```python
from build123d import *


with BuildPart() as part:
    # Sweep1: sweep along a path in Sketch2
    with BuildLine(Plane.XY) as sweep1_path:
        Line((3.4, -33.829572862), (-194.6, -53.729321604))
        ThreePointArc((-194.6, -53.729321604), (-254, 0), (-194.6, 53.729321604))
        Line((-194.6, 53.729321604), (3.4, 33.829572862))
        ThreePointArc((3.4, 33.829572862), (34, 0), (3.4, -33.829572862))
    # Sketch4 → Sweep1 (sweep)
    with BuildSketch(Plane(origin=(0, 0, 0), x_dir=(0, 0, -1), z_dir=(1, 0, 0))):
        Polygon((0, 34.171285719), (6.035, 34.171285719), (9.499101615, 40.171285719), (-9.499101615, 40.171285719), (-6.035, 34.171285719), align=None)
    sweep(path=sweep1_path.line)


solid = part.part
```
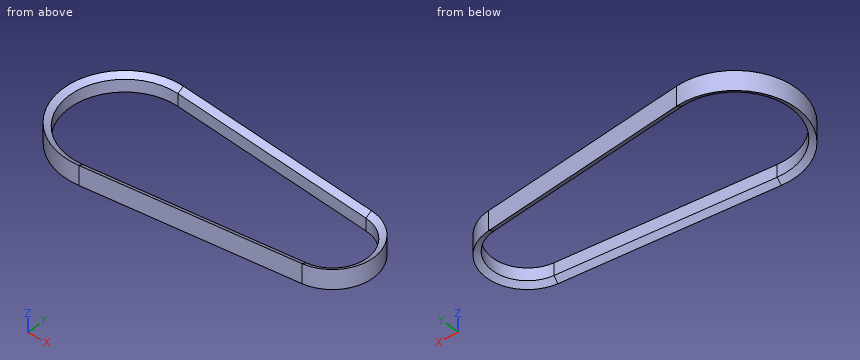
Source: CAD feature listing. Evaluate the final solid. Frame: model axes, mm. Round coordinates to 2 decimals unless told otherwise and drop trailing zeros. Order: outer loops, then holes, each group sorted by start corner. A loop starts at its lowest first (then second) coordinate and runs counter-clockwise, first axis right, second up. Notation, with made-up numbers: (32.25, 74.5) -> (63.25, 74.5) arc R18 ccw to (63.25, 88.5) -> close; hole circle Ø4 at (47.25, 25.5). An arc over 180 degrees is marked (long way). One line per item, written item: value. Start each with the question number.
Q1. Material intervals for probe 1 along Y at (x, z) = (-200, 0); probe 2 along X at (y, z) = (-30, -5); probe 3 along X at (y, z) = (2, 8.75), sorted ascending.
Q2. Section query A-A (z = -2.75). Return the cut outline in (x, y), plus the area to 3 significant figures.
Q3. Pin query (flat end, axial travel): pin 1 (1 mm diameter, centred on x = -15, z = 3.5, fed in from +Y); pin 2 (10 mm diameter, centred on x = 2.5, z = 7.5, fed in from +Y); pin 3 (1 mm diameter, centred on x = -99.5, y = 47, fed in from +Z). Return the tip coordinate at first contact, or that it passes through.
Q4. Section query B-B (x = -39.5). Return the cut outline in (y, z) (3 decimals).
Findings below:
1. probe 1: -59.97 to -54, 54 to 59.97
1. probe 2: -251.93 to -244.9, 16 to 26.42
1. probe 3: -259.94 to -258.65, 38.63 to 39.92
2. outline: (-194.6, 59.73) arc R59.97 ccw (long way) to (-193.41, -59.61) -> (4.59, -39.71) arc R39.97 ccw to (3.4, 39.83) -> close; hole (-194.6, -53.73) -> (3.4, -33.83) arc R34 ccw to (3.4, 33.83) -> (-194.6, 53.73) arc R54 ccw (long way) to start
2. area: 4,160 mm²
3. pin 1: y = 41.73
3. pin 2: y = 40.42
3. pin 3: z = 7.96
4. outline: (-44.141, -9.499) -> (-38.141, -6.035) -> (-38.141, 6.035) -> (-44.141, 9.499) -> close; (38.141, -6.035) -> (44.141, -9.499) -> (44.141, 9.499) -> (38.141, 6.035) -> close
